Could you check a few things on this drawing? It's one solid part, dimensions in mm from its lowest x, y, z. A direction names the side the tool comes from. Round coordinates to 2 decimals unless told otherwise and drop trailing zeros. Order: outer loops, then holes, each group sorted by start corner. A loop starts at its lowest first (then second) coordinate and runs counter-clockwise, first axis right, second up. Notation, with made-up numbers: (-4, 58.25) -> (42, 58.25) arc R31 cw to (42, 91.25) -> close; hole circle Ø10 at (-2, 73.5). An arc over 180 degrees is marked (long way). Use a Markdown table: item, result. Add a question column.
(1) If I drill on probe 1 along X at (y, z) = (7.5, 3.75) (1 decimal); probe 2 along Y at (x, z) = (13.5, 10.25) (1 decimal); probe 3 along Z at (x, y) = (44.5, 3) (1 decimal), over which ranges is the centre line in solid material (lowest first)?
(2) On a 3-axis mill with a long thin cutter (end or side, diameter ignored), from which of +Z, -Z, +X, -X, +Y, -Y can I reach the whole of each face in a straight line? I mean the marked faces 5 and 6. Say none if no direction works.
(3) I want a section at C-C, the plane y = 17.25. Please give me the cut outline in (x, z) (1 decimal).
(4) I'm going to push flat-ended pins straight in: P1, Ø3, axis at x = 45, y = 7, coming from the -Z side (1 decimal); P2, Ø12.5, axis at x = 23.5, y = 7.5, coming from the -Z side; P3, Ø14, axis at x = 38.83, y = 11.27, coming from the -Z side; P4, Ø7, axis at x = 15, z = 17, coming from the -Y side. Where does each tip first touch, or does it pass through?
(5) I want a section at A-A, the plane x = 25.4. Please give me the cut outline in (y, z) (1 decimal).
(6) I want a section at B-B, the plane z = 23.5. Please give me the cut outline in (x, y) (1 decimal).
(7) I want a section at D-D, the plane z = 13.5. Please give me the cut outline in (x, y) (1 decimal).
(8) Thinking about a two-plate mould opening in X: for the marked faces 1, 2, 3 and 4, which applies, pulls with the +X half, pulls with the -X half, needs draft (parallel to the pull), parting line crosses it, or undercut?
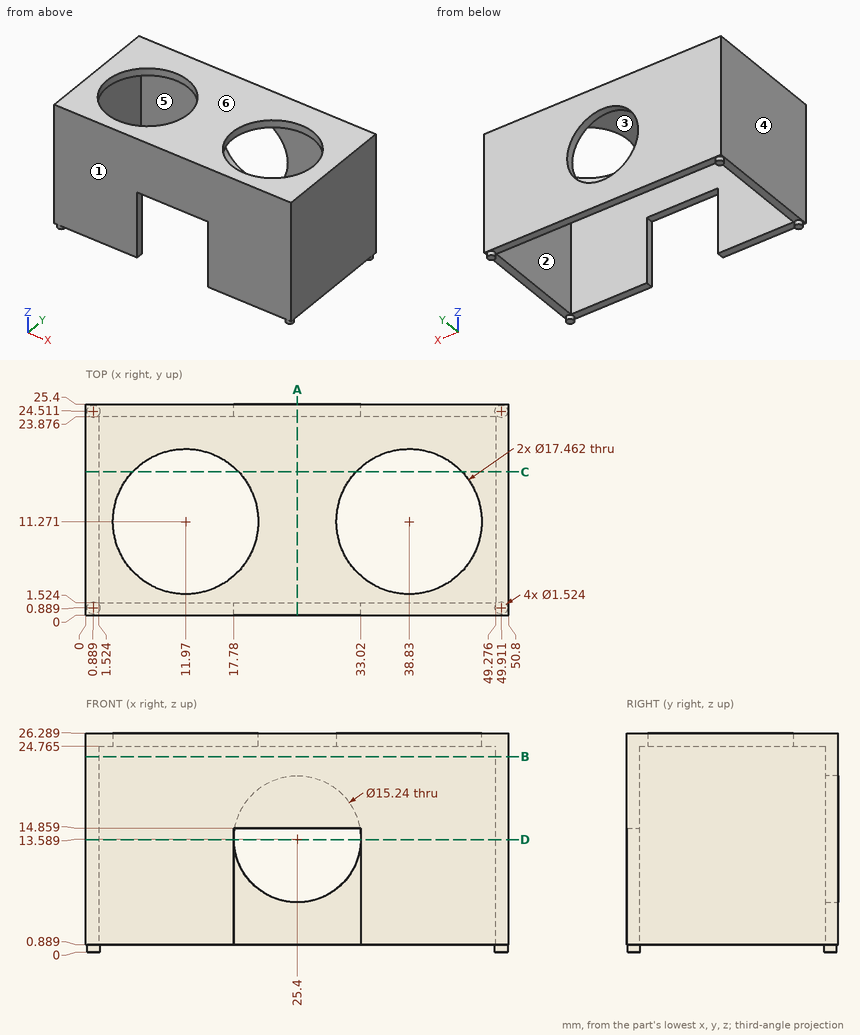
Taken from the geometry:
| question | item | result |
|---|---|---|
| 1 | probe 1 | x = 0 to 1.5, 49.3 to 50.8 |
| 1 | probe 2 | y = 0 to 1.5, 23.9 to 25.4 |
| 1 | probe 3 | z = 24.8 to 26.3 |
| 2 | face 5 | -Z |
| 2 | face 6 | +Z, +X, -X, +Y, -Y |
| 3 | outline | (0, 0.9) -> (1.5, 0.9) -> (1.5, 24.8) -> (5.6, 24.8) -> (5.6, 26.3) -> (0, 26.3) -> close; (18.3, 24.8) -> (32.5, 24.8) -> (32.5, 26.3) -> (18.3, 26.3) -> close; (45.2, 24.8) -> (49.3, 24.8) -> (49.3, 0.9) -> (50.8, 0.9) -> (50.8, 26.3) -> (45.2, 26.3) -> close |
| 4 | P1 | stops at z = 24.8 |
| 4 | P2 | stops at z = 14.86 |
| 4 | P3 | passes through |
| 4 | P4 | stops at y = 0 |
| 5 | outline | (0, 14.9) -> (1.5, 14.9) -> (1.5, 24.8) -> (23.9, 24.8) -> (23.9, 21.2) -> (25.4, 21.2) -> (25.4, 26.3) -> (0, 26.3) -> close; (23.9, 0.9) -> (25.4, 0.9) -> (25.4, 6) -> (23.9, 6) -> close |
| 6 | outline | (0, 0) -> (50.8, 0) -> (50.8, 25.4) -> (0, 25.4) -> close; hole (1.5, 1.5) -> (49.3, 1.5) -> (49.3, 23.9) -> (1.5, 23.9) -> close |
| 7 | outline | (0, 0) -> (17.8, 0) -> (17.8, 1.5) -> (1.5, 1.5) -> (1.5, 23.9) -> (17.8, 23.9) -> (17.8, 25.4) -> (0, 25.4) -> close; (33, 0) -> (50.8, 0) -> (50.8, 25.4) -> (33, 25.4) -> (33, 23.9) -> (49.3, 23.9) -> (49.3, 1.5) -> (33, 1.5) -> close |
| 8 | face 1 | needs draft |
| 8 | face 2 | undercut |
| 8 | face 3 | undercut |
| 8 | face 4 | pulls with the -X half |
